CAD build for the part. Positions are in the model's coordinates, mm. Face numbers are marked on the shaded views. A direction names the side the tool comes from. Coordinates: 2 decimals unless noted, no trailing zeros. Order: outer loops, then holes, each group sorted by start corner. A loop starts at its lowest first (then second) coordinate and runs counter-clockwise, first axis right, second up. Notation, with made-up numbers: (44.5, 18.25) - (50.5, 18.25) arc R14 ccw to (50.5, 25.25) - close; hole circle Ø7 at (-34.5, 37.25). An arc over 180 degrees is marked (long way). Write each question's results on one line, items separated by ' | '. Start each with the question number.
Q1. Which spindle directions (+Z, -Z, +X, -X, +Y, -Y) get a long thin tool onto all of the face, cutting with end or side? Do the marked faces 1 and 2. Say none if no direction does.
Q2. Band-saw the part on A-A, the plane x = -33.5. Write the cut outline in (y, z), then the cut area to 3 significant figures.
Q3. Band-saw the part on D-D, the plane z = 8.25. Write the cut outline in (x, y), then the cut area to 3 significant figures.
Q4. Pin check, flat tips, straight feed: P1, Ø1, axis at y = 27, z = 0.5, coming from the -X side; P2, Ø3, axis at y = -31, z = 3.5, coming from the -X side; P3, Ø5, axis at x = -28.5, y = 7, coming from the -Z side; P4, Ø14.5, axis at x = -11.5, y = -11.5, coming from the +Z side. Stop position of each tip, or through.
Q5. Pull direction Z, two halves, no side cores. Call the marked faces 3, 4, 5 and 6: released by +Z, released by -Z, zero draft, split by the parting line, or undercut.
Q6. Wall check: probe 1 along Y at (x, z) = (-28, 3); probe 2 along Y at (x, z) = (14.5, -0.45); probe 3 along Z at (x, y) = (-33.5, -44). Give the ranges that are in metal, low to high.
Q7. Band-saw the part on B-B, the plane x = -1.5. Write the cut outline in (y, z).
Q8. Band-saw the part on C-C, the plane y = -44. Write the cut outline in (x, z).
```python
from build123d import *

# Parameters (mm, degrees)
BODYS_W                       = 48
BODYS_H                       = 114
BODY_DEPTH                    = 1.7
MIRROR1_START                 = -1.7
MIRROR1_OUTLINE_R             = 4.1
MIRROR1_DEPTH                 = 3.4
KNUCKLEBODY_REACH             = 63.87
KNUCKLEBODY_DIRECTION_2_REACH = 63.87
HOLECHAMFER_SIZE              = 1.4
KNUCKLECUTS_W                 = 17
KNUCKLECUTS_H                 = 24
KNUCKLECUT_DEPTH              = 71.965414111


# Read off the part's stored shape, not the designer's step: Mirror1
with BuildPart() as part:
    # BodyS → Body (new, symmetric)
    with BuildSketch(Plane.XY):
        Rectangle(BODYS_W, BODYS_H)
    extrude(amount=BODY_DEPTH, both=True)

    # Mirror1 outline → Mirror1 (cut)
    with BuildSketch(Plane.XY.offset(MIRROR1_START)):
        with Locations((14.5, 15.5)):
            Circle(MIRROR1_OUTLINE_R)
        with Locations((-1.5, 44)):
            Circle(MIRROR1_OUTLINE_R)
        with Locations((14.5, -15.5)):
            Circle(MIRROR1_OUTLINE_R)
        with Locations((-1.5, -44)):
            Circle(MIRROR1_OUTLINE_R)
    extrude(amount=MIRROR1_DEPTH, mode=Mode.SUBTRACT)

    # KnuckleBody: up to this face of the body (flat: up to its plane)
    knucklebody_end = Plane(part.part.faces().sort_by_distance((0, 57, 0))[0])
    # KnuckleBodyS → KnuckleBody (add, up to the picked face)
    with BuildSketch(Plane(origin=(0, 0, 0), x_dir=(1, 0, 0), z_dir=(0, 1, 0)), mode=Mode.PRIVATE) as knucklebody_sk1:
        with BuildLine():
            Line((-30.783018868, 4.190566038), (-24.724528302, 1.835849057))
            ThreePointArc((-24.724528302, 1.835849057), (-24.36857707, 1.734255626), (-24, 1.7))
            Line((-24, 1.7), (-24, -1.7))
            ThreePointArc((-24, -1.7), (-24.995158089, -1.607509809), (-25.956226415, -1.333207547))
            Line((-25.956226415, -1.333207547), (-32.014716981, 1.021509434))
            ThreePointArc((-32.014716981, 1.021509434), (-37.25246893, -4.451961541), (-29.678490566, -4.285283019))
            Line((-29.678490566, -4.285283019), (-28.555471698, -1.395849057))
            Line((-28.555471698, -1.395849057), (-25.386415094, -2.62754717))
            Line((-25.386415094, -2.62754717), (-26.509433962, -5.516981132))
            ThreePointArc((-26.509433962, -5.516981132), (-40.364272432, -5.821880867), (-30.783018868, 4.190566038))
        make_face()
    knucklebody_tool1 = split(extrude(knucklebody_sk1.sketch, amount=KNUCKLEBODY_REACH, mode=Mode.PRIVATE), bisect_by=knucklebody_end, keep=Keep.BOTH, mode=Mode.PRIVATE)
    add(knucklebody_tool1.solids().sort_by(Axis((-40.156774, 0, 5.730533), (0, 1, 0)))[0])

    # KnuckleBody direction 2: up to this face of the body (flat: up to its plane)
    knucklebody_direction_2_end = Plane(part.part.faces().sort_by_distance((0, -57, 0))[0])
    # KnuckleBodyS → KnuckleBody direction 2 (add, up to the picked face)
    with BuildSketch(Plane(origin=(0, 0, 0), x_dir=(1, 0, 0), z_dir=(0, 1, 0)), mode=Mode.PRIVATE) as knucklebody_direction_2_sk1:
        with BuildLine():
            Line((-30.783018868, 4.190566038), (-24.724528302, 1.835849057))
            ThreePointArc((-24.724528302, 1.835849057), (-24.36857707, 1.734255626), (-24, 1.7))
            Line((-24, 1.7), (-24, -1.7))
            ThreePointArc((-24, -1.7), (-24.995158089, -1.607509809), (-25.956226415, -1.333207547))
            Line((-25.956226415, -1.333207547), (-32.014716981, 1.021509434))
            ThreePointArc((-32.014716981, 1.021509434), (-37.25246893, -4.451961541), (-29.678490566, -4.285283019))
            Line((-29.678490566, -4.285283019), (-28.555471698, -1.395849057))
            Line((-28.555471698, -1.395849057), (-25.386415094, -2.62754717))
            Line((-25.386415094, -2.62754717), (-26.509433962, -5.516981132))
            ThreePointArc((-26.509433962, -5.516981132), (-40.364272432, -5.821880867), (-30.783018868, 4.190566038))
        make_face()
    knucklebody_direction_2_tool1 = split(extrude(knucklebody_direction_2_sk1.sketch, amount=-KNUCKLEBODY_DIRECTION_2_REACH, mode=Mode.PRIVATE), bisect_by=knucklebody_direction_2_end, keep=Keep.BOTH, mode=Mode.PRIVATE)
    add(knucklebody_direction_2_tool1.solids().sort_by(Axis((-40.156774, 0, 5.730533), (0, -1, 0)))[0])

    # HoleChamfer
    holechamfer_edges = [part.edges().sort_by_distance(p)[0] for p in [
        (10.4, 15.5, 1.7),
        (-5.6, 44, 1.7),
        (10.4, -15.5, 1.7),
        (-5.6, -44, 1.7),
    ]]
    chamfer(holechamfer_edges, length=HOLECHAMFER_SIZE)

    # KnuckleCutS → KnuckleCut (cut, symmetric)
    with BuildSketch(Plane.XY):
        with Locations((-32.5, 23)):
            Rectangle(KNUCKLECUTS_W, KNUCKLECUTS_H)
    knucklecut = extrude(amount=KNUCKLECUT_DEPTH, both=True, mode=Mode.SUBTRACT)

    # KCVM: KnuckleCut across plane
    add(knucklecut.mirror(Plane.ZX), mode=Mode.SUBTRACT)


solid = part.part
```
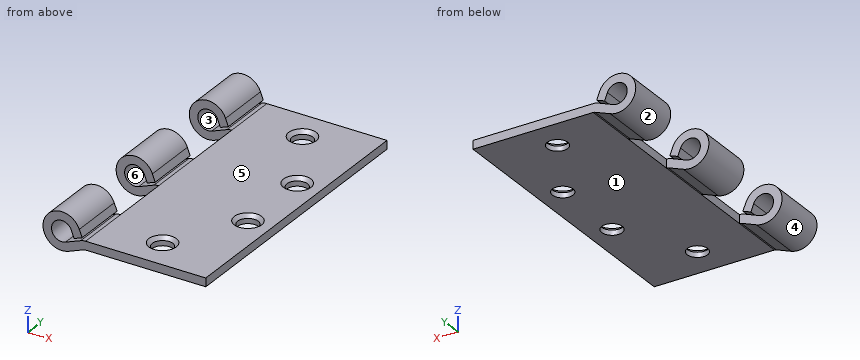
Results below:
1) face 1: -Z, +X, +Y, -Y | face 2: +Y, -Y
2) outline: (-57, -4.7) - (-35, -4.7) - (-35, -1.3) - (-57, -1.3) - close; (-57, 6.9) - (-35, 6.9) - (-35, 10.3) - (-57, 10.3) - close; (-11, -4.7) - (11, -4.7) - (11, -1.3) - (-11, -1.3) - close; (-11, 6.9) - (11, 6.9) - (11, 10.3) - (-11, 10.3) - close; (35, -4.7) - (57, -4.7) - (57, -1.3) - (35, -1.3) - close; (35, 6.9) - (57, 6.9) - (57, 10.3) - (35, 10.3) - close | area: 449 mm²
3) outline: (-38.65, -57) - (-28.35, -57) - (-28.35, -35) - (-38.65, -35) - close; (-38.65, -11) - (-28.35, -11) - (-28.35, 11) - (-38.65, 11) - close; (-38.65, 35) - (-28.35, 35) - (-28.35, 57) - (-38.65, 57) - close | area: 680 mm²
4) P1: stops at x = -24 | P2: passes through | P3: stops at z = -4.27 | P4: stops at z = 1.7
5) face 3: undercut | face 4: split by the parting line | face 5: released by +Z | face 6: undercut
6) probe 1: y = -57 to -35, -11 to 11, 35 to 57 | probe 2: y = -57 to -19.6, -11.4 to 11.4, 19.6 to 57 | probe 3: z = -4.7 to -1.3, 6.9 to 10.3
7) outline: (-57, -1.7) - (-48.1, -1.7) - (-48.1, 0.3) - (-49.5, 1.7) - (-57, 1.7) - close; (-39.9, -1.7) - (39.9, -1.7) - (39.9, 0.3) - (38.5, 1.7) - (-38.5, 1.7) - (-39.9, 0.3) - close; (48.1, -1.7) - (57, -1.7) - (57, 1.7) - (49.5, 1.7) - (48.1, 0.3) - close
8) outline: (-32.01, -1.02) arc R4.1 cw (long way) to (-29.68, 4.29) - (-28.56, 1.4) - (-25.39, 2.63) - (-26.51, 5.52) arc R7.5 ccw (long way) to (-30.78, -4.19) - (-24.72, -1.84) arc R2 cw to (-24, -1.7) - (-5.6, -1.7) - (-5.6, 0.3) - (-7, 1.7) - (-24, 1.7) arc R5.4 ccw to (-25.96, 1.33) - close; (2.6, -1.7) - (24, -1.7) - (24, 1.7) - (4, 1.7) - (2.6, 0.3) - close
